Autodesk Inventor part; units mm, degrees
ref_plane "YZ Plane" through (0, 0, 0) normal (1, 0, 0) x (0, 1, 0)
ref_plane "XZ Plane" through (0, 0, 0) normal (0, 1, 0) x (-1, 0, 0)
ref_plane "XY Plane" through (0, 0, 0) normal (0, 0, 1) x (1, 0, 0)
sketch "Sketch1" plane through (0, 0, 0) normal (0, 0, 1) x (1, 0, 0)
  circle A0 centre (0, 0) radius 3.75
  dimension "d0" = 7.5
extrude "Extrusion1" add sketch "Sketch1" along normal blind 2.3
fillet "Fillet3" radius 0.5 1 edges at (-3.75, 0, 0)
fillet "Fillet4" radius 2.3 1 edges at (-3.75, 0, 2.3)
sketch "草圖6" plane through (0, 0, 2.3) normal (0, 0, 1) x (1, 0, 0)
  circle A0 centre (0, 0) radius 1.505
  line L0 (0.7217, 1.25) -> (1.4434, 0)
  line L1 (1.4434, 0) -> (0.7217, -1.25)
  line L2 (0.7217, -1.25) -> (-0.7217, -1.25)
  line L3 (-0.7217, -1.25) -> (-1.4434, 0)
  line L4 (-1.4434, 0) -> (-0.7217, 1.25)
  line L5 (-0.7217, 1.25) -> (0.7217, 1.25)
  dimension "d27" = 2.5
extrude "擠出4" cut sketch "草圖6" against normal blind 2 contours L0 L1 L2 L3 L4 L5
sketch "草圖7" plane through (0, 0, 0) normal (1, 0, 0) x (0, 1, 0)
  line L0 (0, 0.3) -> (-2, 1.5017)
  line L1 (-2, 1.5017) -> (-2, 0.3)
  line L2 (0, 0.3) -> (-2, 0.3)
  line L3 (0, 0) -> (0, 2.4201)
  dimension "d30" = 0.3
  dimension "d31" = 31
  dimension "d34" = 2
revolve "迴轉3" add sketch "草圖7" angle 360 about axis through (0, 0, 0) along (0, 0, 1)
sketch "草圖8" plane through (0, 0, 0) normal (0, 0, -1) x (-1, 0, 0)
  circle A0 centre (0, 0) radius 3.25
  circle A1 centre (0, 0) radius 2
  dimension "d35" = 4
extrude "擠出5" add sketch "草圖8" along normal blind 8 contours A1
thread "螺紋2"
properties part number "screw_M3_10_hex"
Build history of the part. All positions in model axes, mm. A direction names the side the tool comes from. Coordinates: 2 decimals unless noted, no trailing zeros. Write each loop counter-clockwise with the first axis right and the second up, starting at its lowest first coordinate (ties: lowest second). Pieces come first, ordered by that corner, then holes.
1. Pull direction Y, two halves, no side cores. Call faces 3 (the flat face through (-1.088, 0.616, 1.684)), 4 (the flat face through (0, 0, -8)), 5 (the cylindrical face through (0, 2, -4)): released by +Y, released by -Y, zero draft, split by the parting line, or undercut.
Answer block:
face 3: undercut
face 4: zero draft
face 5: split by the parting line
2. Drop flat-ended pins along their axis: pin 1 (3 mm diameter, centred on x = -1, z = -6.5, fed in from +Y); pin 2 (1 mm diameter, centred on x = 1, y = -2.5, fed in from +Z); pin 3 (1.5 mm diameter, centred on x = 0.5, z = -2, fed in from -Y). Give the stop position or say it passes through.
Answer block:
pin 1: stops at y = 2
pin 2: stops at z = 2.19
pin 3: stops at y = -2
3. Drill centre lines: probe 1 along Z at (x, y) = (0.5, -1.5); probe 2 along Z at (x, y) = (-2.75, 2); probe 3 along X at (y, z) = (1.25, -4.75). Where is each one in solid material? Low to high.
Answer block:
probe 1: z = -8 to 2.3
probe 2: z = 0.02 to 1.3
probe 3: x = -1.56 to 1.56
4. Band-saw the part on A-A, the plane z = -0.5. Give the cut face in (x, y), and give its area (3 significant figures).
Answer block:
outline: circle Ø4 at (0, 0)
area: 12.6 mm2
5. 3-axis set-ups, long thin cutter, end or side, ignore diameter. For faces 1 (the flat face through (1, -2, 0)), 2 (the flat face through (0, 1.25, 2)): which of +Z, -Z, +X, -X, +Y, -Y reach the whole face in a straight line?
Answer block:
face 1: -Z
face 2: +Z
